For this review, take the finished solid that the model builds, in its own axes (mm). Round coordinates to 2 decimals unless told otherwise and drop trailing zeros. Write each loop counter-clockwise with the first axis right and the second up, starting at its lowest first coordinate (ties: lowest second). Pieces come first, ordered by that corner, then holes. Notation, with made-up numbers: (50.5, -27) -> (66.5, -27) arc R29 cw to (66.5, -5) -> close; hole circle Ø10 at (58.5, 77). An arc over 180 degrees is marked (long way). Answer as CSV lines item,"result". Start each with the question number.
Item 1: Take a section at D-D on y = -41. Give the boundary of the cut face in (x, z) (3 decimals).
Item 2: Take a section at C-C on z = 2.1. Count the separate pieces of the cut face and the enclosed holes in it, then the cut area to 3 significant figures.
Item 3: Take a section at A-A on y = 0. Give the boundary of the cut face in (x, z) (3 decimals), then the cut area to 3 significant figures.
Item 4: Wall thickness on probe 1 along X at (y, z) = (8, 0.7) (3 decimals); probe 2 along X at (y, z) = (-2, 1.75) (3 decimals); probe 3 along X at (y, z) = (32, 0.5) (3 decimals): over which ranges is each line inside the solid? List them lowest first. Write a range as from..to.
Item 5: For pin 1 Ø4 at (x, y) = (-67.945, 39.37) entering from +Z; pin 2 Ø1.6 at (y, z) = (58.5, 2) entering from +X; pin 3 Ø4 at (x, y) = (43, -22) entering from -Z; pin 4 Ø2.5 at (x, y) = (-32.46, 31.75) entering from +Z, all flat-tipped, find the tip position at first contact; note any pin that passes through.
Item 6: Take a section at B-B on x = 55. Give the boundary of the cut face in (y, z) (3 decimals), then the cut area to 3 significant figures.
```python
from build123d import *

# Parameters (mm, degrees)
BOSS_EXTRUDE1_DEPTH           = 3.175
MIRROR2_COPY_1_DEPTH          = 3.175
INTERNAL_SHARPS_R             = 9.525
IMU_MOUNTING_DEPTH            = 3.175
IMU_MOUNTING_HOLES_AT_2_COUNT = 2
IMU_MOUNTING_HOLES_AT_2_PITCH = 21.59
IMU_TOOLING_RADIUS_R          = 6.35
SKETCH18_R                    = 4.7625
MCU_MOUNTING_RIBS_DEPTH       = 3.175
TOOLING_RADIUS_R              = 6.35
TOOLING_RADIUS_SMALL_R        = 3.175
SKETCH6_R                     = 6.35
MATERIAL_REMOVAL_DEPTH        = 99.935771608
MCU_MOUNTING_HOLES_AT_2_COUNT = 2
MCU_MOUNTING_HOLES_AT_2_PITCH = 45.72
MCU_MOUNTING_HOLES_AT_3_COUNT = 2
MCU_MOUNTING_HOLES_AT_3_PITCH = 88.57441442
MCU_MOUNTING_HOLES_AT_4_COUNT = 2
MCU_MOUNTING_HOLES_AT_4_PITCH = 75.093140098
MCU_MOUNTING_HOLES_AT_5_COUNT = 2
MCU_MOUNTING_HOLES_AT_5_PITCH = 39.97120776


with BuildPart() as part:
    # Sketch1 → Boss-Extrude1 (new body)
    with BuildSketch(Plane.XY):
        with BuildLine():
            Line((9.434743879, 15.24), (0, 15.24))
            Line((0, 15.24), (0, 0))
            Line((0, 0), (12.7, 0))
            Line((12.7, 0), (12.7, 12.892596045))
            Line((12.7, 12.892596045), (51.712045103, 51.904641149))
            ThreePointArc((51.712045103, 51.904641149), (62.784313673, 54.107052302), (69.05625, 44.720436252))
            Line((69.05625, 44.720436252), (69.05625, 0))
            Line((69.05625, 0), (73.025, 0))
            Line((73.025, 0), (73.025, 57.15))
            Line((73.025, 57.15), (69.85, 57.15))
            Line((69.85, 57.15), (69.85, 60.325))
            ThreePointArc((69.85, 60.325), (65.930039796, 66.191635031), (59.009871939, 64.815128061))
            Line((59.009871939, 64.815128061), (9.434743879, 15.24))
        make_face()
    boss_extrude1 = extrude(amount=BOSS_EXTRUDE1_DEPTH)

    # Sketch11 → CSK for #4 Flat Head Machine Screw1 (revolve, cut)
    with BuildSketch(Plane(origin=(63.5, 60.325, 3.175), x_dir=(0, -1, 0), z_dir=(1, 0, 0))):
        Polygon((0, 0), (0, 3.175), (1.4732, 3.175), (1.4732, 2.030745349), (3.2385, 0), align=None)
    csk_for_4_flat_head_machine_screw1 = revolve(axis=Axis((63.5, 60.325, 9.525), (0, 0, -1)), mode=Mode.SUBTRACT)

    # Mirror1: Boss-Extrude1, CSK for #4 Flat Head Machine Screw1 across plane
    add(boss_extrude1.mirror(Plane.ZX))
    add(csk_for_4_flat_head_machine_screw1.mirror(Plane.ZX), mode=Mode.SUBTRACT)

    # Mirror2: Boss-Extrude1, CSK for #4 Flat Head Machine Screw1 across plane
    add(boss_extrude1.mirror(Plane(origin=(0, 0, 0), x_dir=(0, 0, 1), z_dir=(1, 0, 0))))
    add(csk_for_4_flat_head_machine_screw1.mirror(Plane(origin=(0, 0, 0), x_dir=(0, 0, 1), z_dir=(1, 0, 0))), mode=Mode.SUBTRACT)

    # Mirror2 copy 1 sketch → Mirror2 copy 1 (add)
    with BuildSketch(Plane(origin=(0, 0, 0), x_dir=(-1, 0, 0), z_dir=(0, 0, 1))):
        with BuildLine():
            Line((9.434743879, 15.24), (0, 15.24))
            Line((0, 15.24), (0, 0))
            Line((0, 0), (12.7, 0))
            Line((12.7, 0), (12.7, 12.892596045))
            Line((12.7, 12.892596045), (51.712045103, 51.904641149))
            ThreePointArc((51.712045103, 51.904641149), (62.784313673, 54.107052302), (69.05625, 44.720436252))
            Line((69.05625, 44.720436252), (69.05625, 0))
            Line((69.05625, 0), (73.025, 0))
            Line((73.025, 0), (73.025, 57.15))
            Line((73.025, 57.15), (69.85, 57.15))
            Line((69.85, 57.15), (69.85, 60.325))
            ThreePointArc((69.85, 60.325), (65.930039796, 66.191635031), (59.009871939, 64.815128061))
            Line((59.009871939, 64.815128061), (9.434743879, 15.24))
        make_face()
    extrude(amount=MIRROR2_COPY_1_DEPTH)

    # Mirror2 copy 2 sketch → Mirror2 copy 2 (revolve, cut)
    with BuildSketch(Plane(origin=(-63.5, -60.325, 3.175), x_dir=(0, 1, 0), z_dir=(-1, 0, 0))):
        Polygon((0, 0), (0, 3.175), (1.4732, 3.175), (1.4732, 2.030745349), (3.2385, 0), align=None)
    revolve(axis=Axis((-63.5, -60.325, 9.525), (0, 0, -1)), mode=Mode.SUBTRACT)

    # INTERNAL-SHARPS
    internal_sharps_edges = [part.edges().sort_by_distance(p)[0] for p in [
        (-9.434743879, 15.24, 1.5875),
        (-12.7, 12.892596045, 1.5875),
        (9.434743879, 15.24, 1.5875),
        (12.7, 12.892596045, 1.5875),
        (9.434743879, -15.24, 1.5875),
        (12.7, -12.892596045, 1.5875),
        (-12.7, -12.892596045, 1.5875),
        (-9.434743879, -15.24, 1.5875),
    ]]
    fillet(internal_sharps_edges, radius=INTERNAL_SHARPS_R)

    # Sketch13 → IMU-MOUNTING (add)
    with BuildSketch(Plane.XY):
        with BuildLine():
            Line((-73.025, 44.45), (-73.025, 12.7))
            Line((-73.025, 12.7), (-67.945, 12.7))
            ThreePointArc((-67.945, 12.7), (-62.895851895, 18.339020045), (-69.05625, 22.736967161))
            Line((-69.05625, 22.736967161), (-69.05625, 34.413032839))
            ThreePointArc((-69.05625, 34.413032839), (-62.895851895, 38.810979955), (-67.945, 44.45))
            Line((-67.945, 44.45), (-73.025, 44.45))
        make_face()
    extrude(amount=IMU_MOUNTING_DEPTH)

    # Sketch15 → IMU-MOUNTING-HOLES (revolve, cut)
    with BuildSketch(Plane(origin=(-67.945, 17.78, 3.175), x_dir=(0, -1, 0), z_dir=(1, 0, 0))):
        Polygon((0, 0), (0, 3.175), (1.4732, 3.175), (1.4732, 2.030745349), (3.2385, 0), align=None)
    imu_mounting_holes = revolve(axis=Axis((-67.945, 17.78, 9.525), (0, 0, -1)), mode=Mode.SUBTRACT)

    # IMU-MOUNTING-HOLES at 2: IMU-MOUNTING-HOLES ×2
    with Locations(*[(0, i * IMU_MOUNTING_HOLES_AT_2_PITCH, 0) for i in range(1, IMU_MOUNTING_HOLES_AT_2_COUNT)]):
        add(imu_mounting_holes, mode=Mode.SUBTRACT)

    # IMU-TOOLING-RADIUS
    imu_tooling_radius_edges = [part.edges().sort_by_distance(p)[0] for p in [
        (-69.05625, 44.45, 1.5875),
        (-69.05625, 12.7, 1.5875),
        (-69.05625, 22.736967161, 1.5875),
        (-69.05625, 34.413032839, 1.5875),
    ]]
    fillet(imu_tooling_radius_edges, radius=IMU_TOOLING_RADIUS_R)

    # Sketch18 → MCU-MOUNTING-RIBS (add)
    with BuildSketch(Plane(origin=(0, 0, 0), x_dir=(-1, 0, 0), z_dir=(0, 0, -1))):
        with Locations((8.1788, 17.78)):
            Circle(SKETCH18_R)
        with BuildLine():
            Line((32.4612, -32.653796045), (37.2237, -37.416296045))
            Line((37.2237, -37.416296045), (37.2237, -13.97))
            ThreePointArc((37.2237, -13.97), (35.828796045, -10.602403955), (32.4612, -9.2075))
            Line((32.4612, -9.2075), (9.014903955, -9.2075))
            Line((9.014903955, -9.2075), (13.777403955, -13.97))
            Line((13.777403955, -13.97), (27.6987, -13.97))
            ThreePointArc((27.6987, -13.97), (29.093603955, -17.337596045), (32.4612, -18.7325))
            Line((32.4612, -18.7325), (32.4612, -32.653796045))
        make_face()
        with BuildLine():
            Line((32.4612, 26.9875), (26.794903955, 26.9875))
            Line((26.794903955, 26.9875), (37.2237, 37.416296045))
            Line((37.2237, 37.416296045), (37.2237, 31.75))
            ThreePointArc((37.2237, 31.75), (35.828796045, 28.382403955), (32.4612, 26.9875))
        make_face()
        with BuildLine():
            Line((-42.6212, -10.4775), (-10.284903955, -10.4775))
            Line((-10.284903955, -10.4775), (-15.047403955, -15.24))
            Line((-15.047403955, -15.24), (-37.8587, -15.24))
            ThreePointArc((-37.8587, -15.24), (-39.253603955, -18.607596045), (-42.6212, -20.0025))
            Line((-42.6212, -20.0025), (-42.6212, -42.813796045))
            Line((-42.6212, -42.813796045), (-47.3837, -47.576296045))
            Line((-47.3837, -47.576296045), (-47.3837, -15.24))
            ThreePointArc((-47.3837, -15.24), (-45.988796045, -11.872403955), (-42.6212, -10.4775))
        make_face()
        with BuildLine():
            Line((-42.6212, 28.2575), (-28.064903955, 28.2575))
            Line((-28.064903955, 28.2575), (-47.3837, 47.576296045))
            Line((-47.3837, 47.576296045), (-47.3837, 33.02))
            ThreePointArc((-47.3837, 33.02), (-45.988796045, 29.652403955), (-42.6212, 28.2575))
        make_face()
    extrude(amount=-MCU_MOUNTING_RIBS_DEPTH)

    # TOOLING-RADIUS
    tooling_radius_edges = [part.edges().sort_by_distance(p)[0] for p in [
        (-37.2237, -37.416296045, 1.5875),
        (47.3837, -47.576296045, 1.5875),
        (-26.794903955, 26.9875, 1.5875),
        (-37.2237, 37.416296045, 1.5875),
        (28.064903955, 28.2575, 1.5875),
        (47.3837, 47.576296045, 1.5875),
        (-12.858570933, 18.663827054, 1.5875),
        (-4.150176631, 15.24, 1.5875),
    ]]
    fillet(tooling_radius_edges, radius=TOOLING_RADIUS_R)

    # TOOLING-RADIUS-SMALL
    # the kernel refuses this fillet: 3.175 mm, written as the material it adds along each edge
    with BuildSketch(Plane(origin=(42.6212, -20.0025, 0), x_dir=(-0.9789063129307034, 0.2043096436892193, 0), z_dir=(0, 0, 1)), Plane(origin=(-27.6987, -13.97, 0), x_dir=(-0.2043096436892193, -0.9789063129307034, 0), z_dir=(0, 0, 1))) as tooling_radius_small_piece_1:
        with BuildLine():
            CenterArc((2.594732475, 3.108027544), TOOLING_RADIUS_SMALL_R, 191.789089239, 66.421821522)
            Line((-0.513295069, 2.459344425), (0, 0))
            ThreePointArc((0, 0), (0.973024678, 0.100458685), (1.946049356, 0))
        make_face()
    extrude(amount=3.175)
    with BuildSketch(Plane(origin=(37.8587, -15.24, 0), x_dir=(-1, 0, 0), z_dir=(0, 0, 1)), Plane(origin=(-32.4612, -18.7325, 0), x_dir=(0, -1, 0), z_dir=(0, 0, 1))) as tooling_radius_small_piece_2:
        with BuildLine():
            CenterArc((2.512338916, 3.175), TOOLING_RADIUS_SMALL_R, 203.578178478, 66.421821522)
            ThreePointArc((-0.397596651, 1.905), (-0.100458685, 0.973024678), (0, 0))
            Line((0, 0), (2.512338916, 0))
        make_face()
    extrude(amount=3.175)
    with BuildSketch(Plane(origin=(42.6212, -42.813796045, 0), x_dir=(0, 1, 0), z_dir=(0, 0, 1))) as tooling_radius_small_piece_3:
        with BuildLine():
            CenterArc((TOOLING_RADIUS_SMALL_R * 2.41421356237, TOOLING_RADIUS_SMALL_R), TOOLING_RADIUS_SMALL_R, 135, 135)
            Line((TOOLING_RADIUS_SMALL_R * 1.70710678119, TOOLING_RADIUS_SMALL_R * 1.70710678119), (0, 0))
            Line((0, 0), (TOOLING_RADIUS_SMALL_R * 2.41421356237, 0))
        make_face()
    extrude(amount=3.175)
    with BuildSketch(Plane(origin=(-32.4612, -32.653796045, 0), x_dir=(0, 1, 0), z_dir=(0, 0, 1))) as tooling_radius_small_piece_4:
        with BuildLine():
            CenterArc((TOOLING_RADIUS_SMALL_R * 2.41421356237, -TOOLING_RADIUS_SMALL_R), TOOLING_RADIUS_SMALL_R, 90, 135)
            Line((TOOLING_RADIUS_SMALL_R * 1.70710678119, -TOOLING_RADIUS_SMALL_R * 1.70710678119), (0, 0))
            Line((0, 0), (TOOLING_RADIUS_SMALL_R * 2.41421356237, 0))
        make_face()
    extrude(amount=3.175)
    with BuildSketch(Plane(origin=(-14.131964455, -13.97, 0), x_dir=(-1, 0, 0), z_dir=(0, 0, 1))) as tooling_radius_small_piece_5:
        with BuildLine():
            CenterArc((7.310567561, 3.175), TOOLING_RADIUS_SMALL_R, 135, 135)
            Line((5.06550353, 5.42006403), (4.840997127, 5.644570433))
            ThreePointArc((4.840997127, 5.644570433), (1.133337052, 1.936910358), (-0.269767852, 0.167426271))
            Line((-0.269767852, 0.167426271), (0, -0.3175))
            Line((0, -0.3175), (7.310567561, -0.3175))
            Line((7.310567561, -0.3175), (7.310567561, 0))
        make_face()
    extrude(amount=3.175)
    with BuildSketch(Plane(origin=(15.074724308, -15.24, 0), x_dir=(0.7053179071572191, -0.7088911410388483, 0), z_dir=(0, 0, 1))) as tooling_radius_small_piece_6:
        with BuildLine():
            CenterArc((7.63781192, 3.174989865), TOOLING_RADIUS_SMALL_R, 135.144766988, 135)
            Line((5.387082547, 5.414374221), (5.16200961, 5.638312656))
            Line((5.16200961, 5.638312656), (-0.225072937, 0.223938436))
            Line((-0.225072937, 0.223938436), (-0.019410524, -0.316906108))
            ThreePointArc((-0.019410524, -0.316906108), (0.607184355, -0.33528533), (7.646636273, -0.317498987))
            Line((7.646636273, -0.317498987), (7.645834059, 0))
        make_face()
    extrude(amount=3.175)

    # Sketch6 → MATERIAL-REMOVAL (cut, through all)
    with BuildSketch(Plane(origin=(0, 0, 0), x_dir=(-1, 0, 0), z_dir=(0, 0, -1))):
        Circle(SKETCH6_R)
    extrude(amount=-MATERIAL_REMOVAL_DEPTH, mode=Mode.SUBTRACT)

    # Sketch20 → MCU-MOUNTING-HOLES (revolve, cut)
    with BuildSketch(Plane(origin=(-32.4612, -13.97, 3.175), x_dir=(0, -1, 0), z_dir=(1, 0, 0))):
        Polygon((0, 0), (0, 3.175), (1.4732, 3.175), (1.4732, 2.030745349), (3.2385, 0), align=None)
    mcu_mounting_holes = revolve(axis=Axis((-32.4612, -13.97, 9.525), (0, 0, -1)), mode=Mode.SUBTRACT)

    # MCU-MOUNTING-HOLES at 2: MCU-MOUNTING-HOLES ×2
    with Locations(*[(0, i * MCU_MOUNTING_HOLES_AT_2_PITCH, 0) for i in range(1, MCU_MOUNTING_HOLES_AT_2_COUNT)]):
        add(mcu_mounting_holes, mode=Mode.SUBTRACT)

    # MCU-MOUNTING-HOLES at 3: MCU-MOUNTING-HOLES ×2
    with Locations(*[Vector(0.8476759399659948, 0.5305143737946855, 0) * (i * MCU_MOUNTING_HOLES_AT_3_PITCH) for i in range(1, MCU_MOUNTING_HOLES_AT_3_COUNT)]):
        add(mcu_mounting_holes, mode=Mode.SUBTRACT)

    # MCU-MOUNTING-HOLES at 4: MCU-MOUNTING-HOLES ×2
    with Locations(*[Vector(0.9998569763114565, -0.016912330451817784, 0) * (i * MCU_MOUNTING_HOLES_AT_4_PITCH) for i in range(1, MCU_MOUNTING_HOLES_AT_4_COUNT)]):
        add(mcu_mounting_holes, mode=Mode.SUBTRACT)

    # MCU-MOUNTING-HOLES at 5: MCU-MOUNTING-HOLES ×2
    with Locations(*[Vector(0.6074972801935523, 0.7943217575752515, 0) * (i * MCU_MOUNTING_HOLES_AT_5_PITCH) for i in range(1, MCU_MOUNTING_HOLES_AT_5_COUNT)]):
        add(mcu_mounting_holes, mode=Mode.SUBTRACT)


solid = part.part
```
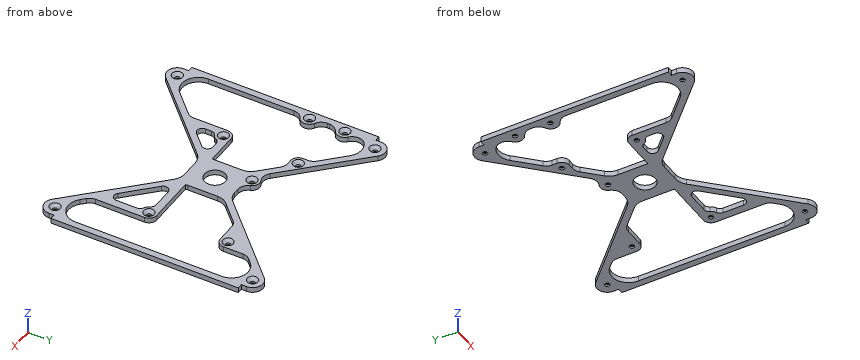
Output values:
1,outline,"(-73.025, 0) -> (-69.056, 0) -> (-69.056, 3.175) -> (-73.025, 3.175) -> close; (-40.807, 0) -> (-35.195, 0) -> (-35.195, 3.175) -> (-40.807, 3.175) -> close; (35.195, 0) -> (47.384, 0) -> (47.384, 3.175) -> (35.195, 3.175) -> close; (69.056, 0) -> (73.025, 0) -> (73.025, 3.175) -> (69.056, 3.175) -> close"
2,separate pieces,"1"
2,enclosed holes,"16"
2,area,"4,070 mm^2"
3,outline,"(-73.025, 0) -> (-69.056, 0) -> (-69.056, 3.175) -> (-73.025, 3.175) -> close; (-12.7, 0) -> (-6.35, 0) -> (-6.35, 3.175) -> (-12.7, 3.175) -> close; (6.35, 0) -> (12.7, 0) -> (12.7, 3.175) -> (6.35, 3.175) -> close; (69.056, 0) -> (73.025, 0) -> (73.025, 3.175) -> (69.056, 3.175) -> close"
3,area,"65.5 mm^2"
4,probe 1,"x = -73.025..-69.045, -12.7..12.7, 69.056..73.025"
4,probe 2,"x = -73.025..-69.056, -12.7..-6.027, 6.027..12.7, 69.056..73.025"
4,probe 3,"x = -73.025..-68.411, -37.224..-33.913, -31.009..-26.195, 26.195..41.558, 43.684..47.273, 69.056..73.025"
5,pin 1,"stops at z = 1.75"
5,pin 2,"stops at x = 69.85"
5,pin 3,"stops at z = 0"
5,pin 4,"passes through"
6,outline,"(-60.805, 0) -> (-54.104, 0) -> (-54.104, 3.175) -> (-60.805, 3.175) -> close; (54.104, 0) -> (60.805, 0) -> (60.805, 3.175) -> (54.104, 3.175) -> close"
6,area,"42.6 mm^2"
